Read the model definition and answer for the solid it produces. Units are mm, in the model's axes. Face numbers are marked on the shaded views. A direction names the side the tool comes from. Coordinates: 2 decimals unless noted, no trailing zeros. Write each loop counter-clockwise with the first axis right and the second up, starting at its lowest first coordinate (ties: lowest second). Pieces come first, ordered by that corner, then holes.
Autodesk Inventor part; units mm, degrees
ref_plane "YZ Plane" through (0, 0, 0) normal (1, 0, 0) x (0, 1, 0)
ref_plane "XZ Plane" through (0, 0, 0) normal (0, 1, 0) x (-1, 0, 0)
ref_plane "XY Plane" through (0, 0, 0) normal (0, 0, 1) x (1, 0, 0)
sketch "Sketch1" plane through (0, 0, 0) normal (0, 1, 0) x (-1, 0, 0)
  circle A0 centre (0, 0) radius 3.2
  circle A1 centre (0, 0) radius 3.4
  circle A2 centre (0, 0) radius 5
  circle A3 centre (0, 0) radius 6
  line L0 (0, 0) -> (0, -15)
  line L1 (0, 0) -> (0, 15)
  line L2 (0, 0) -> (-9, 0)
  circle A4 centre (-9, 0) radius 3.75
  line L3 (0, 15) -> (0, 6)
  line L4 (0, 6) -> (10, 6)
  line L5 (10, 6) -> (10, 15)
  line L6 (10, 15) -> (0, 15)
  line L7 (10, 10.5) -> (5, 10.5)
  line L8 (0, -15) -> (10, -15)
  line L9 (10, -15) -> (10, -6)
  line L10 (10, -6) -> (0, -6)
  line L11 (10, -10.5) -> (5, -10.5)
  circle A5 centre (5, 10.5) radius 2.5
  circle A6 centre (5, -10.5) radius 2.5
  line L12 (0, -6) -> (-30, -6)
  line L13 (-30, -6) -> (-30, 6)
  line L14 (-30, 6) -> (0, 6)
  line L15 (0, 15) -> (-30, 15)
  line L16 (-30, 15) -> (-30, 6)
  line L17 (0, -15) -> (-30, -15)
  line L18 (-30, -15) -> (-30, -6)
  line L19 (-35, 0) -> (-41, 0)
  line L20 (-41, 0) -> (-30, -15)
  line L21 (-41, 0) -> (-30, 15)
  circle A7 centre (-35, 0) radius 2.5
  dimension "d3" = 12
  dimension "d0" = 6.4
  dimension "d1" = 6.8
  dimension "d2" = 10
  dimension "d4" = 15
  dimension "d5" = 15
  dimension "d6" = 9
  dimension "d7" = 7.5
  dimension "d8" = 10
  dimension "d9" = 5
  dimension "d10" = 10
  dimension "d11" = 10
  dimension "d12" = 5
  dimension "d13" = 5
  dimension "d14" = 5
  dimension "d15" = 30
  dimension "d17" = 6
  dimension "d18" = 5
extrude "Extrusion1" add sketch "Sketch1" along normal blind 3 contours L1 L6 L5 L4 | L10 L9 L8 L0 | L13 L18 L20 L21 L16
extrude "Extrusion2" add sketch "Sketch1" along normal blind 15 contours L14 L16 L15 L1 | L0 L17 L18 L12
sketch "Sketch2" plane through (-10, 0, 15) normal (0, 0, 1) x (1, 0, 0)
  line L0 (10, 15) -> (10, 7.5)
  line L1 (10, 3) -> (10, 15)
  line L2 (10, 7.5) -> (17, 7.5)
  arc A0 (17, 12) -> (17, 3) centre (17, 7.5) ccw
  line L3 (17, 7.5) -> (40, 7.5)
  line L4 (40, 3) -> (40, 15)
  line L5 (40, 7.5) -> (33, 7.5)
  arc A1 (33, 3) -> (33, 12) centre (33, 7.5) ccw
  line L6 (17, 3) -> (33, 3)
  line L7 (17, 12) -> (33, 12)
  point P0 (10, 0)
  dimension "d23" = 7.5
  dimension "d24" = 7
  dimension "d25" = 9
  dimension "d26" = 7
  dimension "d27" = 9
extrude "Extrusion3" cut sketch "Sketch2" against normal blind 31
properties part number "push_clip(1)"
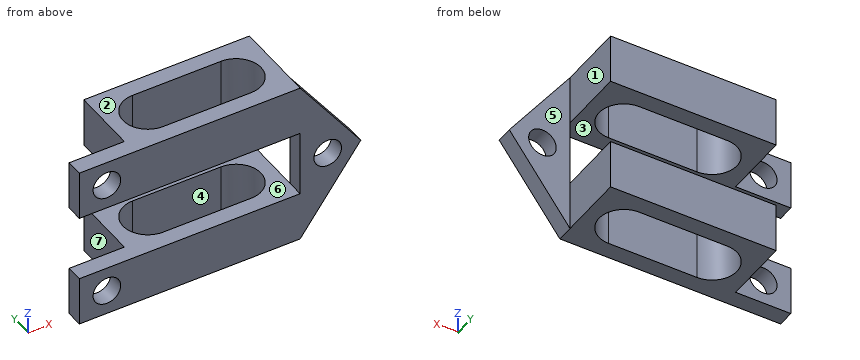
Item 1: For the marked faces 4, 5, 6 and 7, determine the directions among +Z, -Z, +X, -X, +Y, -Y from which every point of the face is accessible in a straight line to the end or side of a thin tool.
Item 2: The part is cut by section A-A (z = -10.5). Give the vertices of the cut face in (x, y).
Item 3: The part is cut by section D-D (x = 7.5). Give the vertices of the cut face in (y, z), and give its area (3 significant figures).
Item 4: The part is cut by section B-B (y = 7.5). Give the vertices of the cut face in (x, z).
Item 5: Determine the mould class of the marked faces 1, 2 and 3 for opening direction Z: +Z half, -Z half, draft (parallel to the pull), parting line (faces both ways), or undercut.
Item 6: Find the intervals of material crossed by probe 1 along Z at (x, y) = (-5, 0.6); probe 2 along Z at (x, y) = (16, 2.25); probe 3 along X at (y, z) = (1.65, 0), in increasing order.
Item 7: Given pin 1 (3 mm diameter, centred on x = 35, z = 0, fed in from +Y); pin 2 (7 mm diameter, centred on y = 10.5, z = 11.5, fed in from +X); pin 3 (10 mm diameter, centred on x = 17, z = -10, fed in from -Y); pin 4 (6.5 mm diameter, centred on x = -5, z = -10.5, fed in from +Y), each flat-ended and moving along its own axis, determine where each tip first touches the part or whether it passes through.
Item 8: The part is cut by section C-C (x = 29). Give the vertices of the cut face in (y, z), and give its area (3 significant figures).
Answer:
1. face 4: +Z, -Z
1. face 5: +Z, -Z, +X, +Y
1. face 6: -X, +Y, -Y
1. face 7: +Z, -Z, -X, +Y
2. outline: (-10, 0) - (-7.5, 0) - (-7.5, 3) - (-10, 3) - close; (-2.5, 0) - (33.3, 0) - (33.3, 3) - (30, 3) - (30, 15) - (0, 15) - (0, 3) - (-2.5, 3) - close; hole (7, 3) - (23, 3) arc R4.5 ccw to (23, 12) - (7, 12) arc R4.5 ccw to start
3. outline: (0, -15) - (3, -15) - (3, -6) - (0, -6) - close; (0, 6) - (3, 6) - (3, 15) - (0, 15) - close; (12, -15) - (15, -15) - (15, -6) - (12, -6) - close; (12, 6) - (15, 6) - (15, 15) - (12, 15) - close
3. area: 108 mm2
4. outline: (0, -15) - (2.5, -15) - (2.5, -6) - (0, -6) - close; (0, 6) - (2.5, 6) - (2.5, 15) - (0, 15) - close; (27.5, -15) - (30, -15) - (30, -6) - (27.5, -6) - close; (27.5, 6) - (30, 6) - (30, 15) - (27.5, 15) - close
5. face 1: draft
5. face 2: +Z half
5. face 3: undercut
6. probe 1: z = -15 to -13, -8 to -6, 6 to 8, 13 to 15
6. probe 2: z = -15 to -6, 6 to 15
6. probe 3: x = 30 to 32.5, 37.5 to 41
7. pin 1: passes through
7. pin 2: stops at x = 30
7. pin 3: stops at y = 0
7. pin 4: stops at y = 3
8. outline: (0, -15) - (15, -15) - (15, -6) - (0, -6) - close; (0, 6) - (15, 6) - (15, 15) - (0, 15) - close
8. area: 270 mm2
